Verification items for the finished model (mm, model axes). Face numbers are marked on the shaded views. A direction names the side the tool comes from. Coordinates: 2 decimals unless noted, no trailing zeros. Order: outer loops, then holes, each group sorted by start corner. A loop starts at its lowest first (then second) coordinate and runs counter-clockwise, first axis right, second up.
Q1. Cross-section at C-C, the plane x = 37.5. Record the boundary of the cut face in (y, z), and give its area (3 significant figures).
Q2. Depth check by flat-ended pin: P1, Ø4, axis at x = -1, z = -31, coming from the +Y side; P2, Ø1.5, axis at x = -48.5, y = 14.5, coming from the +Z side; P3, Ø0.8, axis at x = 47, z = 36, coming from the +Y side. Enter the tip coordinate at first touch or a pass-through.
Q3. Draft check along Z on the marked faces 3, 4, 5 and 6. Enter one of: pulls with the +Z half, pulls with the -Z half, needs draft (parallel to the pull), parting line crosses it, or undercut.
Q4. Cross-section at A-A, the plane y = 5.5. Record the boundary of the cut face in (x, z), and give its area (3 significant figures).
Q5. Cross-section at D-D, the plane z = 28. Record the boundary of the cut face in (x, y), and give its area (3 significant figures).
Q6. Set-up check for the marked faces 1 and 2: record each of +Z, -Z, +X, -X, +Y, -Y from which the full face is reachable in a straight line by a thin tool's end or side.
Q7. Cross-section at B-B, the plane z = 0. Record the boundary of the cut face in (x, y).
Q8. Thickness scan on line 1 (X direction, y = 11, z = -20.5); line 2 (Z direction, x = 33.5, y = 7.5); line 3 (Z direction, x = -46, y = 32). Record the ranges inside material, lowest first.
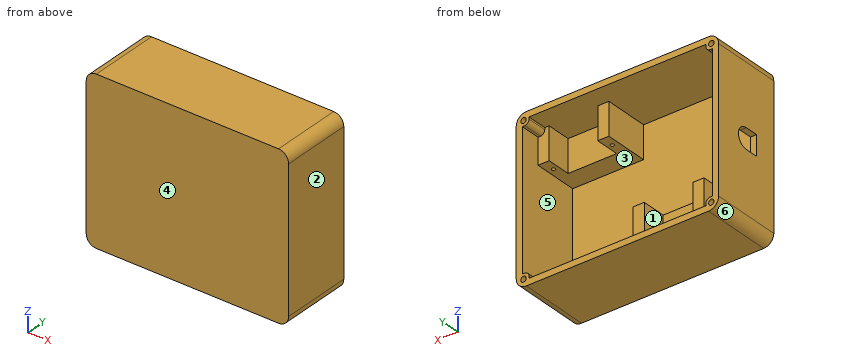
from build123d import *

# Parameters (mm, degrees)
EXTRUDE_1_DEPTH     = 35
SHELL_2_T           = -3
EXTRUDE_3_DEPTH     = 32
SKETCH_3_R          = 1.35
CUT_EXTRUDE_1_DEPTH = 4
CUT_EXTRUDE_4_DEPTH = 3
SKETCH_7_W          = 35
SKETCH_7_H          = 21
SKETCH_7_H_2        = 16
EXTRUDE_4_DEPTH     = 22
SKETCH_8_W          = 24
SKETCH_8_H          = 16
CUT_EXTRUDE_5_DEPTH = 12
SKETCH_9_R          = 0.9
CUT_EXTRUDE_6_DEPTH = 5
SKETCH_10_R         = 0.9
CUT_EXTRUDE_7_DEPTH = 4


with BuildPart() as part:
    # 草图1 → 凸台-拉伸1 (new body)
    with BuildSketch(Plane(origin=(0, 0, 0), x_dir=(1, 0, 0), z_dir=(0, 1, 0))):
        with BuildLine():
            Line((-45, 40), (45, 40))
            ThreePointArc((45, 40), (48.535533906, 38.535533906), (50, 35))
            Line((50, 35), (50, -35))
            ThreePointArc((50, -35), (48.535533906, -38.535533906), (45, -40))
            Line((45, -40), (-45, -40))
            ThreePointArc((-45, -40), (-48.535533906, -38.535533906), (-50, -35))
            Line((-50, -35), (-50, 35))
            ThreePointArc((-50, 35), (-48.535533906, 38.535533906), (-45, 40))
        make_face()
    extrude(amount=EXTRUDE_1_DEPTH)

    # 抽壳2
    shell_2_openings = [part.faces().sort_by_distance(p)[0] for p in [
        (0, 35, 0),
    ]]
    offset(amount=SHELL_2_T, openings=shell_2_openings, kind=Kind.INTERSECTION)

    # 草图2 → 凸台-拉伸3 (add)
    with BuildSketch(Plane(origin=(0, 3, 0), x_dir=(1, 0, 0), z_dir=(0, 1, 0))):
        with BuildLine():
            Line((47, 33.834963516), (47, 35))
            ThreePointArc((47, 35), (46.414213562, 36.414213562), (45, 37))
            Line((45, 37), (43.678814145, 37))
            Line((43.678814145, 37), (43.678814145, 36))
            ThreePointArc((43.678814145, 36), (44.31293865, 34.46908802), (45.843850629, 33.834963516))
            Line((45.843850629, 33.834963516), (47, 33.834963516))
        make_face()
        with BuildLine():
            Line((-43.678814145, 36), (-43.678814145, 37))
            Line((-43.678814145, 37), (-45, 37))
            ThreePointArc((-45, 37), (-46.414213562, 36.414213562), (-47, 35))
            Line((-47, 35), (-47, 33.834963516))
            Line((-47, 33.834963516), (-45.843850629, 33.834963516))
            ThreePointArc((-45.843850629, 33.834963516), (-44.31293865, 34.46908802), (-43.678814145, 36))
        make_face()
        with BuildLine():
            Line((43.678814145, -37), (45, -37))
            ThreePointArc((45, -37), (46.414213562, -36.414213562), (47, -35))
            Line((47, -35), (47, -33.834963516))
            Line((47, -33.834963516), (45.843850629, -33.834963516))
            ThreePointArc((45.843850629, -33.834963516), (44.31293865, -34.46908802), (43.678814145, -36))
            Line((43.678814145, -36), (43.678814145, -37))
        make_face()
        with BuildLine():
            Line((-47, -33.834963516), (-47, -35))
            ThreePointArc((-47, -35), (-46.414213562, -36.414213562), (-45, -37))
            Line((-45, -37), (-43.678814145, -37))
            Line((-43.678814145, -37), (-43.678814145, -36))
            ThreePointArc((-43.678814145, -36), (-44.31293865, -34.46908802), (-45.843850629, -33.834963516))
            Line((-45.843850629, -33.834963516), (-47, -33.834963516))
        make_face()
    extrude(amount=EXTRUDE_3_DEPTH)

    # 草图3 → 切除-拉伸1 (cut)
    with BuildSketch(Plane(origin=(0, 35, 0), x_dir=(1, 0, 0), z_dir=(0, 1, 0))):
        with Locations((-46.4, 36.4)):
            Circle(SKETCH_3_R)
        with Locations((46.4, 36.4)):
            Circle(SKETCH_3_R)
        with Locations((46.4, -36.4)):
            Circle(SKETCH_3_R)
        with Locations((-46.4, -36.4)):
            Circle(SKETCH_3_R)
    extrude(amount=-CUT_EXTRUDE_1_DEPTH, mode=Mode.SUBTRACT)

    # 草图6 → 切除-拉伸4 (cut)
    with BuildSketch(Plane.ZY.offset(50)):
        with BuildLine():
            Line((-5, 17.418982567), (-5, 10.918982567))
            Line((-5, 10.918982567), (5, 10.918982567))
            Line((5, 10.918982567), (5, 17.418982567))
            ThreePointArc((5, 17.418982567), (0, 22.418982567), (-5, 17.418982567))
        make_face()
    extrude(amount=-CUT_EXTRUDE_4_DEPTH, mode=Mode.SUBTRACT)

    # 草图7 → 凸台-拉伸4 (add)
    with BuildSketch(Plane(origin=(0, 3, 0), x_dir=(1, 0, 0), z_dir=(0, 1, 0))):
        with Locations((-17.5, 26.5)):
            Rectangle(SKETCH_7_W, SKETCH_7_H)
        with Locations((29.5, -29)):
            Rectangle(SKETCH_7_W, SKETCH_7_H_2)
    extrude(amount=EXTRUDE_4_DEPTH)

    # 草图8 → 切除-拉伸5 (cut)
    with BuildSketch(Plane(origin=(0, 25, 0), x_dir=(1, 0, 0), z_dir=(0, 1, 0))):
        with Locations((29.5, -29)):
            Rectangle(SKETCH_8_W, SKETCH_8_H)
        with Locations((-17.5, 24)):
            Rectangle(SKETCH_8_W, SKETCH_8_H)
    extrude(amount=-CUT_EXTRUDE_5_DEPTH, mode=Mode.SUBTRACT)

    # 草图9 → 切除-拉伸6 (cut)
    with BuildSketch(Plane.XY.offset(-16)):
        with Locations((-2.75, 19)):
            Circle(SKETCH_9_R)
        with Locations((-32.25, 19)):
            Circle(SKETCH_9_R)
    extrude(amount=-CUT_EXTRUDE_6_DEPTH, mode=Mode.SUBTRACT)

    # 草图10 → 切除-拉伸7 (cut)
    with BuildSketch(Plane(origin=(0, 0, 21), x_dir=(-1, 0, 0), z_dir=(0, 0, -1))):
        with Locations((-44, 19)):
            Circle(SKETCH_10_R)
        with Locations((-15, 19)):
            Circle(SKETCH_10_R)
    extrude(amount=-CUT_EXTRUDE_7_DEPTH, mode=Mode.SUBTRACT)


solid = part.part
Check values:
1. outline: (0, -40) - (35, -40) - (35, -37) - (3, -37) - (3, 21) - (13, 21) - (13, 37) - (35, 37) - (35, 40) - (0, 40) - close
1. area: 592 mm2
2. P1: stops at y = 25
2. P2: stops at z = 39.18
2. P3: stops at y = 31
3. face 3: undercut
3. face 4: needs draft
3. face 5: undercut
3. face 6: pulls with the -Z half
4. outline: (-50, -35) arc R5 ccw to (-45, -40) - (45, -40) arc R5 ccw to (50, -35) - (50, 35) arc R5 ccw to (45, 40) - (-45, 40) arc R5 ccw to (-50, 35) - close; hole (-47, -33.83) - (-45.84, -33.83) arc R2.17 cw to (-43.68, -36) - (-43.68, -37) - (-35, -37) - (-35, -16) - (0, -16) - (0, -37) - (43.68, -37) - (43.68, -36) arc R2.17 cw to (45.84, -33.83) - (47, -33.83) - (47, 21) - (12, 21) - (12, 37) - (-43.68, 37) - (-43.68, 36) arc R2.17 cw to (-45.84, 33.83) - (-47, 33.83) - close
4. area: 2,350 mm2
5. outline: (-50, 0) - (50, 0) - (50, 35) - (47, 35) - (47, 25) - (41.5, 25) - (41.5, 13) - (17.5, 13) - (17.5, 25) - (12, 25) - (12, 3) - (-47, 3) - (-47, 35) - (-50, 35) - close
5. area: 974 mm2
6. face 1: +Y
6. face 2: +Z, -Z, +X, +Y, -Y
7. outline: (-50, 0) - (50, 0) - (50, 35) - (47, 35) - (47, 3) - (-47, 3) - (-47, 10.92) - (-50, 10.92) - close; (-50, 22.42) - (-47, 22.42) - (-47, 35) - (-50, 35) - close
8. line 1: x = -50 to -47, -35 to 0, 47 to 50
8. line 2: z = -40 to -37, 21 to 40
8. line 3: z = -39.9 to -37.69, -35.11 to -33.83, 33.83 to 35.11, 37.69 to 39.9
